Design review of the part built by this model. Coordinates are the model's own, in mm. Round coordinates to 2 decimals unless told otherwise and drop trailing zeros. Loops run counter-clockwise (first coordinate to the right, second up) from the corner with the lowest first, then second, coordinate; pieces in that order, holes last. Notation, with made-up numbers: M 81.25,-13 L 113.25,-13 A20 cw 113.25,-2 Z; hole C -30.5,23 d7. An arc over 180 degrees is marked long. Use a Markdown table: item, result.
from build123d import *

# Parameters (mm, degrees)
SKETCH1_R           = 100
SKETCH1_R_2         = 4
BOSS_EXTRUDE1_DEPTH = 4
CUT_EXTRUDE2_START  = -4
CUT_EXTRUDE2_DEPTH  = 5
CIRPATTERN14_COUNT  = 4


with BuildPart() as part:
    # Sketch1 → Boss-Extrude1 (new body)
    with BuildSketch(Plane.XY):
        Circle(SKETCH1_R)
        Circle(SKETCH1_R_2, mode=Mode.SUBTRACT)
    extrude(amount=BOSS_EXTRUDE1_DEPTH)

    # Sketch2 → Cut-Extrude2 (cut)
    with BuildSketch(Plane.XY.offset(4).offset(CUT_EXTRUDE2_START)):
        with BuildLine():
            Line((-15, 682.376448842), (-15, 134.079674161))
            Line((-15, 134.079674161), (-15, 60))
            ThreePointArc((-15, 60), (0, 45), (15, 60))
            Line((15, 60), (15, 143.343079639))
            Line((15, 143.343079639), (15, 691.63985432))
            Line((15, 691.63985432), (-308.533757453, 1739.42004133))
            Line((-308.533757453, 1739.42004133), (-338.533757453, 1730.156635852))
            Line((-338.533757453, 1730.156635852), (-15, 682.376448842))
        make_face()
    cut_extrude2 = extrude(amount=CUT_EXTRUDE2_DEPTH, mode=Mode.SUBTRACT)

    # CirPattern14: Cut-Extrude2 ×4 about axis
    cirpattern14_axis = Axis((0, 0, 0), (0, 0, 1))
    for i in range(1, CIRPATTERN14_COUNT):
        add(cut_extrude2.rotate(cirpattern14_axis, i * 360 / CIRPATTERN14_COUNT), mode=Mode.SUBTRACT)


solid = part.part
1. Wall thickness on line 1 along Y through (x, z) = (0, 2.5); line 2 along Y through (x, z) = (-68, 2.2); line 3 along X through (y, z) = (57, 2.6): over which ranges is each line inside the solid? List them lowest first. Write a range as from..to.
Check values:
| item | result |
|---|---|
| line 1 | y = -45..-4, 4..45 |
| line 2 | y = -73.32..-15, 15..73.32 |
| line 3 | x = -82.16..-14.7, 14.7..82.16 |
2. Take a section at D-D on x = -32. Give the boundary of the cut face in (y, z), and give its area (3 significant figures).
Check values:
| item | result |
|---|---|
| outline | M -94.74,0 L 94.74,0 L 94.74,4 L -94.74,4 Z |
| area | 758 mm² |
3. Take a section at A-A on x = 0. Give the boundary of the cut face in (y, z).
Check values:
| item | result |
|---|---|
| outline | M -45,0 L -4,0 L -4,4 L -45,4 Z; M 4,0 L 45,0 L 45,4 L 4,4 Z |
4. The part is to be moulded in two halves that separate along Y. For faces 1 (the face through (45, 0, 2)), 2 (the face through (-45, 0, 2)), 3 (the face through (-1, -21, 4)), 4 (the face through (0, 45, 2)), say which applies: pulls with the +Y half, pulls with the -Y half, needs draft (parallel to the pull), parting line crosses it, or undercut.
Check values:
| item | result |
|---|---|
| face 1 | undercut |
| face 2 | undercut |
| face 3 | needs draft |
| face 4 | pulls with the +Y half |
5. Insertion check: pin 1 (3 mm diameter, centred on x = -12, y = 75.5, fed in from -Z); pin 2 (2 mm diameter, centred on x = 86.5, z = 2, fed in from +Y); pin 3 (1.2 mm diameter, centred on y = -77.5, z = 2, fed in from -X); pin 4 (1.5 mm diameter, centred on x = 75.5, z = 1, fed in from -Y). Each pin has a flat end and moves straight along its axis. Give the tip position at first contact, or say it passes through.
Check values:
| item | result |
|---|---|
| pin 1 | passes through |
| pin 2 | stops at y = 51.86 |
| pin 3 | stops at x = -63.92 |
| pin 4 | stops at y = -66.43 |
6. Take a section at B-B on z = 2.2. Give the boundary of the cut face in (x, y), and give its area (3 significant figures).
Check values:
| item | result |
|---|---|
| outline | M -98.87,-15 A100 ccw -15,-98.87 L -15,-60 A15 cw 15,-60 L 15,-98.87 A100 ccw 98.87,-15 L 60,-15 A15 cw 60,15 L 98.87,15 A100 ccw 15,98.87 L 15,60 A15 cw -15,60 L -15,98.87 A100 ccw -98.87,15 L -60,15 A15 cw -60,-15 Z; hole C 0,0 d8 |
| area | 25,200 mm² |
